from build123d import *

# Parameters (mm, degrees)
SKETCH1_R                      = 15.958
SHAFTHOLDERNEARMOTOR_DEPTH     = 1
SKETCH2_R                      = 3.4
CUT_EXTRUDE1_DEPTH             = 16.85
SKETCH10_R                     = 50
BOSS_EXTRUDE4_DEPTH            = 20
SKETCH12_R                     = 47.082764373
SKETCH12_R_2                   = 15.95790089
CUTTOREMVEEXCESSMATERIAL_DEPTH = 17
SKETCH13_R                     = 50
SKETCH13_R_2                   = 47.082764373
BOSS_EXTRUDE5_DEPTH            = 17
SKETCH32_R                     = 7.75
CUT_EXTRUDE2_DEPTH             = 22


with BuildPart() as part:
    # Sketch1 → ShaftHolderNearMotor (new body)
    with BuildSketch(Plane(origin=(0, 0, 0), x_dir=(1, 0, 0), z_dir=(0, 1, 0))):
        Circle(SKETCH1_R)
    extrude(amount=SHAFTHOLDERNEARMOTOR_DEPTH)

    # Sketch2 → Cut-Extrude1 (cut)
    with BuildSketch(Plane(origin=(0, 1, 0), x_dir=(1, 0, 0), z_dir=(0, 1, 0))):
        Circle(SKETCH2_R)
    extrude(amount=-CUT_EXTRUDE1_DEPTH, mode=Mode.SUBTRACT)

    # Sketch10 → Boss-Extrude4 (add)
    with BuildSketch(Plane.XZ):
        Circle(SKETCH10_R)
    extrude(amount=BOSS_EXTRUDE4_DEPTH)

    # Sketch12 → CutToRemveExcessMaterial (cut)
    with BuildSketch(Plane(origin=(0, 0, 0), x_dir=(1, 0, 0), z_dir=(0, 1, 0))):
        Circle(SKETCH12_R)
        Circle(SKETCH12_R_2, mode=Mode.SUBTRACT)
    extrude(amount=-CUTTOREMVEEXCESSMATERIAL_DEPTH, mode=Mode.SUBTRACT)

    # Sketch13 → Boss-Extrude5 (add)
    with BuildSketch(Plane(origin=(0, 0, 0), x_dir=(1, 0, 0), z_dir=(0, 1, 0))):
        Circle(SKETCH13_R)
        Circle(SKETCH13_R_2, mode=Mode.SUBTRACT)
    extrude(amount=BOSS_EXTRUDE5_DEPTH)

    # Sketch32 → Cut-Extrude2 (cut, through all)
    with BuildSketch(Plane(origin=(0, 1, 0), x_dir=(1, 0, 0), z_dir=(0, 1, 0))):
        Circle(SKETCH32_R)
    extrude(amount=-CUT_EXTRUDE2_DEPTH, mode=Mode.SUBTRACT)


solid = part.part
Geometry: final body of the model. Coordinates: model frame, mm. A direction names the side the tool comes from. Give positions to 0.01 mm unless a question says otherwise; leave off trailing zeros. Order: outer loops, then holes, each group sorted by start corner. A loop starts at its lowest first (then second) coordinate and runs counter-clockwise, first axis right, second up. Notation, with made-up numbers: (-14.5, 17.25) -> (26.5, 17.25) arc R27 cw to (26.5, 49.25) -> close; hole circle Ø1 at (36, 54). An arc over 180 degrees is marked (long way). Write each question's results on one line, items separated by ' | '.
1) First-contact query: pin 1 Ø1.5 at (x, y) = (-3.5, -1) entering from -Z; pin 2 Ø5 at (y, z) = (6, 4.5) entering from -X; pin 3 Ø3 at (y, z) = (-10, 6) entering from +X. Flat tips, straight axial feed; report the tip coordinate or a pass-through.
Geometry says:
pin 1: stops at z = -49.92 | pin 2: stops at x = -49.96 | pin 3: stops at x = 49.8
2) Line query: line 1 along X through (y, z) = (-4.25, 0); line 2 along X through (y, z) = (10, 0). Output: solid intervals per line, ascending.
Geometry says:
line 1: x = -50 to -47.08, -15.96 to -7.75, 7.75 to 15.96, 47.08 to 50 | line 2: x = -50 to -47.08, 47.08 to 50
3) Set-up query: faces 1 (the face through (15.22, -8.38, -4.79)), 2 (the face through (-1, -20, -10)). Return all of +Z, -Z, +X, -X, +Y, -Y with unobstructed straight access to the full face (end or side cutting, diameter ignored); none if empty.
Geometry says:
face 1: +Y | face 2: +Z, -Z, +X, -X, -Y
4) Draft query along Z for faces 3 (the face through (-34, 17, 33)), 4 (the face through (-2.08, 0.49, -15.82)), 5 (the face through (44.91, -0.24, -14.14)), 6 (the face through (47.69, -1.76, -15.02)). Return one class per face: released by +Z, released by -Z, zero draft, split by the parting line, or undercut.
Geometry says:
face 3: zero draft | face 4: undercut | face 5: undercut | face 6: split by the parting line
5) Cut plane C-C (y = 10). Output: boundary loops of the cut face in (x, z), and give its area (3 significant figures).
Geometry says:
outline: circle Ø100 at (0, 0); hole circle Ø94.17 at (0, 0) | area: 890 mm²
